Part model, mm, in its own coordinate system. A direction names the side the tool comes from. Give positions to 0.01 mm unless a question says otherwise; leave off trailing zeros. Order: outer loops, then holes, each group sorted by start corner. A loop starts at its lowest first (then second) coordinate and runs counter-clockwise, first axis right, second up.
1. Drop flat-ended pins along their axis: pin 1 Ø0.5 at (x, y) = (0.5, -6.5) entering from -Z; pin 2 Ø0.8 at (y, z) = (-6.5, -1.5) entering from +X; pin 3 Ø1.5 at (x, y) = (-29.5, -5.5) entering from -Z. Give the stop position or say it passes through.
2. Which spindle directions (+Z, -Z, +X, -X, +Y, -Y) get a long thin tool onto all of the face, cutting with end or side? Do faces 1 (the cylindrical face through (-36.341, -5.574, -0.903)), 2 (the cylindrical face through (31.99, -6.24, 66.6)), 3 (the cylindrical face through (0.42, -4.5, -69.95)). Say none if no direction does.
3. Mould opens along Z. For faces 4 (the cylindrical face through (0.42, -5.57, -71)), 5 (the cylindrical face through (-31.943, -6.24, 66.645)), 6 (the cylindrical face through (-0.42, -5.57, 71)) say: +Z half, -Z half, draft (parallel to the pull), parting line (faces both ways), or undercut.
4. Slice it at A-A on z = -8. List the corners of the cut face in (x, y) (3 decimals).
5. Probe line 1 (Z direction, x = 16, y = -1.75); line 2 (X direction, y = -1.25, z = -59.5) (3 decimals); line 3 (X direction, y = -3.75, z = 14.5). List the from-to ranges inside material, lowest first.
6. Slice it at B-B on x = -28. List the corners of the cut face in (y, z), and give its area (3 significant figures).
from build123d import *

# Parameters (mm, degrees)
F1_DEPTH = 5.11
F2_R     = 5
F3_DEPTH = 7
F4_R     = 5
F5_T     = -1.5


# Not quite as in the source:
# - a shell that OpenCascade refuses in one call is made with other operations: the cavity is built on its own and cut out


with BuildPart() as f1:
    # F0 (on Front) → F1 (new body)
    with BuildSketch(Plane.XZ):
        with BuildLine():
            Line((28.845, 71.765), (-28.845, 71.765))
            ThreePointArc((-28.845, 71.765), (-34.5018542495, 69.4218542495), (-36.845, 63.765))
            Line((-36.845, 63.765), (-36.845, -63.765))
            ThreePointArc((-36.845, -63.765), (-34.5018542495, -69.4218542495), (-28.845, -71.765))
            Line((-28.845, -71.765), (28.845, -71.765))
            ThreePointArc((28.845, -71.765), (34.5018542495, -69.4218542495), (36.845, -63.765))
            Line((36.845, -63.765), (36.845, 63.765))
            ThreePointArc((36.845, 63.765), (34.5018542495, 69.4218542495), (28.845, 71.765))
        make_face()
    extrude(amount=F1_DEPTH)

    # F2
    f2_edges = [f1.edges().sort_by_distance(p)[0] for p in [
        (36.845, -5.11, 0),
    ]]
    fillet(f2_edges, radius=F2_R)

    # F0 (on Front) → F3 (join)
    with BuildSketch(Plane.XZ):
        with BuildLine():
            Line((29.845, 72.5), (-29.845, 72.5))
            ThreePointArc((-29.845, 72.5), (-35.5018542495, 70.1568542495), (-37.845, 64.5))
            Line((-37.845, 64.5), (-37.845, -64.5))
            ThreePointArc((-37.845, -64.5), (-35.5018542495, -70.1568542495), (-29.845, -72.5))
            Line((-29.845, -72.5), (29.845, -72.5))
            ThreePointArc((29.845, -72.5), (35.5018542495, -70.1568542495), (37.845, -64.5))
            Line((37.845, -64.5), (37.845, 64.5))
            ThreePointArc((37.845, 64.5), (35.5018542495, 70.1568542495), (29.845, 72.5))
        make_face()
        with BuildLine():
            ThreePointArc((-36.845, 63.765), (-34.5018542495, 69.4218542495), (-28.845, 71.765))
            Line((-28.845, 71.765), (28.845, 71.765))
            ThreePointArc((28.845, 71.765), (34.5018542495, 69.4218542495), (36.845, 63.765))
            Line((36.845, 63.765), (36.845, -63.765))
            ThreePointArc((36.845, -63.765), (34.5018542495, -69.4218542495), (28.845, -71.765))
            Line((28.845, -71.765), (-28.845, -71.765))
            ThreePointArc((-28.845, -71.765), (-34.5018542495, -69.4218542495), (-36.845, -63.765))
            Line((-36.845, -63.765), (-36.845, 63.765))
        make_face(mode=Mode.SUBTRACT)
        with BuildLine():
            Line((28.845, 71.765), (-28.845, 71.765))
            ThreePointArc((-28.845, 71.765), (-34.5018542495, 69.4218542495), (-36.845, 63.765))
            Line((-36.845, 63.765), (-36.845, -63.765))
            ThreePointArc((-36.845, -63.765), (-34.5018542495, -69.4218542495), (-28.845, -71.765))
            Line((-28.845, -71.765), (28.845, -71.765))
            ThreePointArc((28.845, -71.765), (34.5018542495, -69.4218542495), (36.845, -63.765))
            Line((36.845, -63.765), (36.845, 63.765))
            ThreePointArc((36.845, 63.765), (34.5018542495, 69.4218542495), (28.845, 71.765))
        make_face()
    extrude(amount=F3_DEPTH)

    # F4
    f4_edges = [f1.edges().sort_by_distance(p)[0] for p in [
        (37.845, -7, 0),
    ]]
    fillet(f4_edges, radius=F4_R)

    # F5: a shell. OpenCascade refuses it in one call, so the cavity is built on its own and cut out:
    # the body offset inwards by the wall thickness, plus a prism from it out through each open face.
    f5_core = offset(f1.part, amount=F5_T, kind=Kind.INTERSECTION, mode=Mode.PRIVATE)
    f5_exits = [f5_core.faces().sort_by_distance(p)[0] for p in [
        (0, -1.5, 0),
        (0, -5.5, 0),
    ]]
    add(f5_core, mode=Mode.SUBTRACT)
    extrude(f5_exits, amount=-F5_T, mode=Mode.SUBTRACT)


solid = f1.part
Data:
1. pin 1: stops at z = -70.13
1. pin 2: stops at x = 35.71
1. pin 3: stops at z = -71.68
2. face 1: +Z, -Z, -X, -Y
2. face 2: +Y, -Y
2. face 3: +Y
3. face 4: -Z half
3. face 5: undercut
3. face 6: +Z half
4. outline: (-37.845, -2) arc R5 ccw to (-32.845, -7) - (-32.845, -5.5) arc R3.5 cw to (-36.345, -2) - (-36.345, 0) - (-37.845, 0) - close; (32.845, -7) arc R5 ccw to (37.845, -2) - (37.845, 0) - (36.345, 0) - (36.345, -2) arc R3.5 cw to (32.845, -5.5) - close
5. line 1: z = -72.5 to -71, 71 to 72.5
5. line 2: x = -37.845 to -36.345, 36.345 to 37.845
5. line 3: x = -37.53 to -35.88, 35.88 to 37.53
6. outline: (-7, -67.5) arc R5 ccw to (-2, -72.5) - (0, -72.5) - (0, -71) - (-2, -71) arc R3.5 cw to (-5.5, -67.5) - close; (-7, 67.5) - (-5.5, 67.5) arc R3.5 cw to (-2, 71) - (0, 71) - (0, 72.5) - (-2, 72.5) arc R5 ccw to start
6. area: 26.0 mm2
